Could you check a few things on this model? Use its own coordinates, in mm. A direction names the side the tool comes from. Coordinates: 2 decimals unless noted, no trailing zeros. Loops run counter-clockwise (first coordinate to the right, second up) from the corner with the lowest first, then second, coordinate; pieces in that order, holes last.
from build123d import *

# Parameters (mm, degrees)
BOSS_EXTRUDE1_DEPTH = 6.858
CUT_EXTRUDE1_DEPTH  = 26.4
BOSS_EXTRUDE2_DEPTH = 6.858
SKETCH6_W           = 1.27
SKETCH6_H           = 3.81
CUT_EXTRUDE2_DEPTH  = 6.35


with BuildPart() as part:
    # Sketch1 → Boss-Extrude1 (new body)
    with BuildSketch(Plane(origin=(0, 0, 0), x_dir=(1, 0, 0), z_dir=(0, 1, 0))):
        with BuildLine():
            Line((0, -22.86), (0, -25.4))
            Line((0, -25.4), (12.7, -25.4))
            Line((12.7, -25.4), (12.7, -22.86))
            ThreePointArc((12.7, -22.86), (11.43, -19.05), (12.7, -15.24))
            Line((12.7, -15.24), (12.7, 0))
            Line((12.7, 0), (0, 0))
            Line((0, 0), (0, -15.24))
            ThreePointArc((0, -15.24), (1.27, -19.05), (0, -22.86))
        make_face()
    extrude(amount=BOSS_EXTRUDE1_DEPTH)

    # Sketch2 → Cut-Extrude1 (cut, through all)
    with BuildSketch(Plane.XY.offset(25.4)):
        Polygon((3.048, 0), (3.048, 2.286), (2.032, 2.286), (2.032, 4.826), (5.715, 4.826), (5.715, 1.016), (6.985, 1.016), (6.985, 4.826), (10.668, 4.826), (10.668, 2.286), (9.652, 2.286), (9.652, 0), align=None)
    extrude(amount=-CUT_EXTRUDE1_DEPTH, mode=Mode.SUBTRACT)

    # Sketch5 → Boss-Extrude2 (add, through all)
    with BuildSketch(Plane(origin=(0, 6.858, 0), x_dir=(1, 0, 0), z_dir=(0, 1, 0))):
        with BuildLine():
            Line((0, 0), (0, -2.286))
            ThreePointArc((0, -2.286), (-4.445, -6.731), (0, -11.176))
            Line((0, -11.176), (0, -13.462))
            ThreePointArc((0, -13.462), (-6.731, -6.731), (0, 0))
        make_face()
        with BuildLine():
            Line((12.7, -13.462), (12.7, -11.176))
            ThreePointArc((12.7, -11.176), (17.145, -6.731), (12.7, -2.286))
            Line((12.7, -2.286), (12.7, 0))
            ThreePointArc((12.7, 0), (19.431, -6.731), (12.7, -13.462))
        make_face()
    extrude(amount=-BOSS_EXTRUDE2_DEPTH)

    # Sketch6 → Cut-Extrude2 (cut)
    with BuildSketch(Plane(origin=(0, 0, 0), x_dir=(-1, 0, 0), z_dir=(0, 0, -1))):
        with Locations((-6.35, 2.921)):
            Rectangle(SKETCH6_W, SKETCH6_H)
    extrude(amount=-CUT_EXTRUDE2_DEPTH, mode=Mode.SUBTRACT)


solid = part.part
(1) Which directions (+Z, -Z, +X, -X, +Y, -Y) give clear straight access to the entire face, cutting with the end or side of a thin tool? Please do faces 1 (the face through (12.7, 3, 7)), 2 (the face through (10, 2.286, 13)), 3 (the face through (6, 1.016, 16)).
Answers:
face 1: +Y, -Y
face 2: +Z, -Z
face 3: +Z, -Z, -Y
(2) Imagine slicing it at A-A, the plane x = 2.5. Write out the boundary of the cut face in (y, z), and give its area (3 significant figures).
Answers:
outline: (0, 0) - (2.29, 0) - (2.29, 25.4) - (0, 25.4) - close; (4.83, 0) - (6.86, 0) - (6.86, 25.4) - (4.83, 25.4) - close
area: 110 mm2
(3) Imagine slicing it at B-B, the plane y = 0.5. Write out the boundary of the cut face in (x, z) (3 decimals), and give its area (3 significant figures).
Answers:
outline: (0, 0) - (3.048, 0) - (3.048, 25.4) - (0, 25.4) - (0, 22.86) arc R6.35 cw to (0, 15.24) - (0, 13.462) arc R6.731 ccw to start; (9.652, 0) - (12.7, 0) arc R6.731 ccw to (12.7, 13.462) - (12.7, 15.24) arc R6.35 cw to (12.7, 22.86) - (12.7, 25.4) - (9.652, 25.4) - close; hole (0, 2.286) - (0, 11.176) arc R4.445 ccw to start; hole (12.7, 2.286) arc R4.445 ccw to (12.7, 11.176) - close
area: 222 mm2
(4) Imagine slicing it at C-C, the plane y = 5.5. Write out the boundary of the cut face in (x, z) (3 decimals).
Answers:
outline: (0, 0) - (12.7, 0) arc R6.731 ccw to (12.7, 13.462) - (12.7, 15.24) arc R6.35 cw to (12.7, 22.86) - (12.7, 25.4) - (0, 25.4) - (0, 22.86) arc R6.35 cw to (0, 15.24) - (0, 13.462) arc R6.731 ccw to start; hole (0, 2.286) - (0, 11.176) arc R4.445 ccw to start; hole (12.7, 2.286) arc R4.445 ccw to (12.7, 11.176) - close
(5) For pin 1 (1.1 mm diameter, centred on y = 1.5, z = 18.5, fed in from +X); pin 2 (1.8 mm diameter, centred on y = 1, z = 17, fed in from -X); pin 3 (2.5 mm diameter, centred on x = 7, z = 9.5, fed in from -Y); pin 4 (6 mm diameter, centred on x = -2.5, z = 20, fed in from -Y), each with a flat end and sliding along its axis, tell me the tip position at first contact or that it passes through.
Answers:
pin 1: stops at x = 11.53
pin 2: stops at x = 0.54
pin 3: stops at y = 1.02
pin 4: passes through
(6) Imagine slicing it at D-D, the plane z = 10. Write out the boundary of the cut face in (x, y) (3 decimals), and give its area (3 significant figures).
Answers:
outline: (-5.884, 0) - (-3.012, 0) - (-3.012, 6.858) - (-5.884, 6.858) - close; (0, 0) - (3.048, 0) - (3.048, 2.286) - (2.032, 2.286) - (2.032, 4.826) - (5.715, 4.826) - (5.715, 1.016) - (6.985, 1.016) - (6.985, 4.826) - (10.668, 4.826) - (10.668, 2.286) - (9.652, 2.286) - (9.652, 0) - (12.7, 0) - (12.7, 6.858) - (0, 6.858) - close; (15.712, 0) - (18.584, 0) - (18.584, 6.858) - (15.712, 6.858) - close
area: 94.3 mm2
(7) We'd pull the mould along X, two halves only. Please class faces 4 (the face through (10.668, 4, 13)), 5 (the face through (6, 5, 0)), 6 (the face through (-6.73, 3.48, 6.88)), 7 (the face through (11.43, 3.38, 19.11)): +X half, -X half, draft (parallel to the pull), parting line (faces both ways), or undercut.
Answers:
face 4: undercut
face 5: draft
face 6: -X half
face 7: +X half
(8) I need wall thicknesses on probe 1 along X at (y, z) = (4.5, 18.25) (3 decimals); probe 2 along X at (y, z) = (6, 6.75); probe 3 along Y at (x, z) = (10, 11.75). Which ranges of each line are inside material? Lowest first, please.
Answers:
probe 1: x = 1.219 to 2.032, 5.715 to 6.985, 10.668 to 11.481
probe 2: x = -6.73 to -4.44, 0 to 12.7, 17.14 to 19.43
probe 3: y = 0 to 2.29, 4.83 to 6.86
